Verification items for the finished model (mm, model axes). Face numbers are marked on the shaded views. Round coordinates to 2 decimals unless told otherwise and drop trailing zeros. Order: outer loops, then holes, each group sorted by start corner. A loop starts at its lowest first (then second) coordinate and runs counter-clockwise, first axis right, second up. Notation, with made-up numbers: (-23, 59.25) -> (-16, 59.25) arc R19 ccw to (-16, 66.25) -> close; hole circle Ø4 at (50, 27). An arc over 180 degrees is marked (long way). Answer in a Markdown table with one row per item. Add a question column.
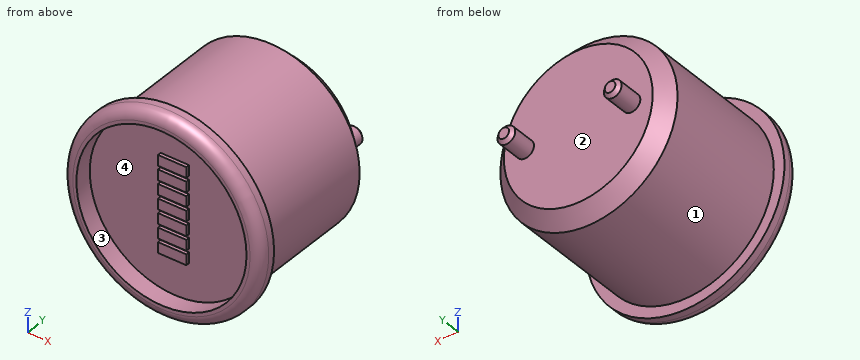
Solid Edge part; units mm, degrees
sketch "Sketch1" plane through (0, 0, 0) normal (0, -1, 0) x (1, 0, 0)
  circle A0 centre (-29.6968, 31.8389) radius 12.5
extrude "Protrusion1" add sketch "Sketch1" against normal blind 20
chamfer "Chamfer_1" distance 2 angle 45 1 edges at (-42.1968, 20, 31.8389)
sketch "Sketch2" plane through (-29.6968, 0, 31.8389) normal (0, -1, 0) x (1, 0, 0)
  circle A0 centre (0, 0) radius 14
  circle A1 centre (0, 0) radius 12
extrude "ExtrudedProtrusion_2" add sketch "Sketch2" along normal blind 2.5
fillet "Round_1" radius 1.5 1 edges at (-43.6968, -2.5, 31.8389)
sketch "Sketch3" plane through (-29.6968, 20, 31.8389) normal (0, 1, 0) x (1, 0, 0)
  circle A0 centre (7.5, 0) radius 1.25
  circle A1 centre (-7.5, 0) radius 1.25
extrude "ExtrudedProtrusion_3" add sketch "Sketch3" along normal blind 4
chamfer "Chamfer_2" distance 0.5 angle 45 2 edges at (-23.4468, 24, 31.8389) (-38.4468, 24, 31.8389)
sketch "Sketch4" plane through (-29.6968, 0, 31.8389) normal (0, -1, 0) x (-1, 0, 0)
  line L0 (-2, -1.2639) -> (2, -1.2639)
  line L1 (2, -1.2639) -> (2, -2.7639)
  line L2 (2, -2.7639) -> (-2, -2.7639)
  line L3 (-2, -2.7639) -> (-2, -1.2639)
  line L4 (-2, -3.2639) -> (2, -3.2639)
  line L5 (2, -3.2639) -> (2, -4.7639)
  line L6 (2, -4.7639) -> (-2, -4.7639)
  line L7 (-2, -4.7639) -> (-2, -3.2639)
  line L8 (-2, -5.2639) -> (2, -5.2639)
  line L9 (2, -5.2639) -> (2, -6.7639)
  line L10 (2, -6.7639) -> (-2, -6.7639)
  line L11 (-2, -6.7639) -> (-2, -5.2639)
  line L12 (-2, 2.75) -> (2, 2.75)
  line L13 (2, 2.75) -> (2, 1.25)
  line L14 (2, 1.25) -> (-2, 1.25)
  line L15 (-2, 1.25) -> (-2, 2.75)
  line L16 (-2, 4.75) -> (2, 4.75)
  line L17 (2, 4.75) -> (2, 3.25)
  line L18 (2, 3.25) -> (-2, 3.25)
  line L19 (-2, 3.25) -> (-2, 4.75)
  line L20 (-2, 6.75) -> (2, 6.75)
  line L21 (2, 6.75) -> (2, 5.25)
  line L22 (2, 5.25) -> (-2, 5.25)
  line L23 (-2, 5.25) -> (-2, 6.75)
  line L24 (-2, 0.75) -> (2, 0.75)
  line L25 (2, 0.75) -> (2, -0.75)
  line L26 (2, -0.75) -> (-2, -0.75)
  line L27 (-2, -0.75) -> (-2, 0.75)
  dimension "D1" = 2
  dimension "D2" = 2
extrude "ExtrudedProtrusion_4" add sketch "Sketch4" along normal blind 0.5
1) Draft check along Z on the marked faces 1, 2, 3 and 4. Enter one of: +Z half, -Z half, draft (parallel to the pull), parting line (faces both ways), or undercut.
2) Cross-section at A-A, the plane y = 22. Record the boundary of the cut face in (x, z).
3) Thickness scan on L1, parallel to Y at x = -29, z = 30.5; L2, parallel to Y at x = -21.75, z = 27; L3, parallel to X at y = 12.75, z = 31.5. Record the ranges inside material, lowest first. Write a range as [from, to].
4) Depth check by flat-ended pin: P1, Ø0.6, axis at x = -28.5, y = -0.5, coming from the -Z side; P2, Ø1.6, axis at x = -30.5, z = 30, coming from the -Y side; P3, Ø8, axis at y = 13.5, z = 26, coming from the +X side. Enter the tip coordinate at first touch or a pass-through.
5) Cross-section at B-B, the plane y = 6.25. Record the boundary of the cut face in (x, z).
Results below:
| question | item | result |
|---|---|---|
| 1 | face 1 | parting line |
| 1 | face 2 | draft |
| 1 | face 3 | undercut |
| 1 | face 4 | undercut |
| 2 | outline | circle Ø2.5 at (-37.2, 31.84); circle Ø2.5 at (-22.2, 31.84) |
| 3 | L1 | [-0.5, 20] |
| 3 | L2 | [0, 20] |
| 3 | L3 | [-42.19, -17.2] |
| 4 | P1 | z = 17.87 |
| 4 | P2 | y = -0.5 |
| 4 | P3 | x = -17.33 |
| 5 | outline | circle Ø25 at (-29.7, 31.84) |
